Geometry: final body of the model. Coordinates: model frame, mm. A direction names the side the tool comes from. Round coordinates to 2 decimals unless told otherwise and drop trailing zeros. Write each loop counter-clockwise with the first axis right and the second up, starting at its lowest first coordinate (ties: lowest second). Pieces come first, ordered by that corner, then holes. Notation, with made-up numbers: M 65.25,-5.75 L 85.25,-5.75 A26 cw 85.25,17.25 Z; hole C 68,44.5 d3. An arc over 180 degrees is marked long. Answer as CSV lines item,"result". Start each with the question number.
Q1. Section query A-A on y = -38. Output: boundary loops of the cut face in (x, z), and give its area (3 significant figures).
Q2. Mould query, pull axis X, two halves, no side actions, for faces 3 (the cylindrical face through (18.783, -0.661, 5.037)), 4 (the flat face through (0, -1, -6)), 5 (the flat face through (-5.08, -1, -8)). Classes: pulls with the +X half, pulls with the -X half, needs draft (parallel to the pull), parting line crosses it, or undercut.
Q3. Ray query, probe 1 along Y at (x, z) = (-46.5, -3); probe 2 along Z at (x, y) = (-28, 38); probe 3 along Y at (x, z) = (-25, -7.5). Return the intervals inside material, ascending.
Q4. Reachability of faces 1 (the flat face through (-131, -96.52, 1)), 2 (the flat face through (-125, 101.6, 2)) from +Z, -Z, +X, -X, +Y, -Y: full face, straight path, thin tool, end or side. Return the list, or none.
Q5. Section query B-B on y = 0. Output: boundary loops of the cut face in (x, z), and give its area (3 significant figures).
Q6. First-contact query: pin 1 (2 mm diameter, centred on x = -151, y = 44, fed in from +Z); pin 2 (8 mm diameter, centred on x = -267.5, y = 29.5, fed in from -Z); pin 3 (1.5 mm diameter, centred on x = -265.5, y = -12, fed in from -Z). Flat tips, straight axial feed; report the tip coordinate or a pass-through.
```python
from build123d import *

# Parameters (mm, degrees)
F2_DEPTH     = 101.6
F3_T         = -5.08
F0_R         = 5.08
F4_DEPTH     = 38.1
F5_T4_DEPTH  = 134.2759536589
F5_S5_R      = 576.6246219757
F5_T6_DEPTH  = 71
F5_T10_DEPTH = 134.2759536589
F5_S11_R     = 576.6246219757
F5_T12_DEPTH = 71
F5_T13_DEPTH = 202.727744005
F6_R         = 12.7
F7_R         = 5.08


# Not quite as in the source:
# - a fillet or chamfer that OpenCascade refuses, or shapes differently, is made with other operations: its cross-section is extruded or revolved along the edge and cut away or added


with BuildPart() as f2:
    # F1 (on Front) → F2 (new body, symmetric)
    with BuildSketch(Plane.XZ):
        with BuildLine():
            Line((0, -49.880515784), (0, 25.847228221))
            Line((0, 25.847228221), (-304.8, 25.847228221))
            ThreePointArc((-304.8, 25.847228221), (-157.6074099904, -32.9761822695), (0, -49.880515784))
        make_face()
    extrude(amount=F2_DEPTH, both=True)

    # F3
    f3_openings = [f2.faces().sort_by_distance(p)[0] for p in [
        (-152.4, 0, 25.847228),
    ]]
    offset(amount=F3_T, openings=f3_openings)

    # F0 (on Right) → F4 (join)
    with BuildSketch(Plane.YZ):
        Circle(F0_R)
    extrude(amount=F4_DEPTH)

    # F5: fillet of radius 25.4 on 4 edges, made by hand


with BuildPart() as f5_tool2:
    # F5_s3 → F5_t4 (new body)
    with BuildSketch(Plane.XY.offset(25.847228221)):
        with BuildLine():
            ThreePointArc((-5.08, -71.12), (-12.5194877579, -89.0805122421), (-30.48, -96.52))
            Line((-30.48, -96.52), (-5.08, -96.52))
            Line((-5.08, -96.52), (-5.08, -71.12))
        make_face()
    extrude(amount=-F5_T4_DEPTH)

    # F5_s5 → F5_t6 (intersect, symmetric)
    with BuildSketch(Plane.XZ.offset(83.8)):
        with Locations((-17.3467118203, 531.5654050176)):
            Circle(F5_S5_R)
    extrude(amount=F5_T6_DEPTH, both=True, mode=Mode.INTERSECT)


with BuildPart() as f2_1:
    add(f2.part)

    # F5_t1: union F5_tool2
    add(f5_tool2.part)


with BuildPart() as f5_tool8:
    # F5_s9 → F5_t10 (new body)
    with BuildSketch(Plane.XY.offset(25.847228221)):
        with BuildLine():
            ThreePointArc((-30.48, 96.52), (-12.5194877579, 89.0805122421), (-5.08, 71.12))
            Line((-5.08, 71.12), (-5.08, 96.52))
            Line((-5.08, 96.52), (-30.48, 96.52))
        make_face()
    extrude(amount=-F5_T10_DEPTH)

    # F5_s11 → F5_t12 (intersect, symmetric)
    with BuildSketch(Plane.XZ.offset(-83.8)):
        with Locations((-17.3467118203, 531.5654050176)):
            Circle(F5_S11_R)
    extrude(amount=F5_T12_DEPTH, both=True, mode=Mode.INTERSECT)


with BuildPart() as f2_2:
    add(f2_1.part)

    # F5_t7: union F5_tool8
    add(f5_tool8.part)

    # F5_s14 → F5_t13 (cut)
    with BuildSketch(Plane.XY.offset(-113.380515784)):
        with BuildLine():
            ThreePointArc((0, -76.2), (-7.4394877579, -94.1605122421), (-25.4, -101.6))
            Line((-25.4, -101.6), (0, -101.6))
            Line((0, -101.6), (0, -76.2))
        make_face()
        with BuildLine():
            ThreePointArc((0, 76.2), (-7.4394877579, 94.1605122421), (-25.4, 101.6))
            Line((-25.4, 101.6), (0, 101.6))
            Line((0, 101.6), (0, 76.2))
        make_face()
    extrude(amount=F5_T13_DEPTH, mode=Mode.SUBTRACT)

    # F6
    f6_edges = [f2_2.edges().sort_by_distance(p)[0] for p in [
        (-7.439388, -94.160412, -50.054842),
        (0, 0, -49.880516),
        (-169.899659, -101.6, -29.779289),
        (-5.918318, 92.497978, -50.026943),
        (-169.899659, 101.6, -29.779289),
    ]]
    fillet(f6_edges, radius=F6_R)

    # F7
    f7_edges = [f2_2.edges().sort_by_distance(p)[0] for p in [
        (-166.679144, -96.52, -25.386819),
        (-10.998525, -87.418225, -45.024272),
        (-5.08, 0, -44.928725),
        (-11.01893, 87.442584, -45.024496),
        (-166.679144, 96.52, -25.386819),
    ]]
    fillet(f7_edges, radius=F7_R)


solid = f2_2.part
```
Entries:
1,outline,"M -304.8,25.85 A581.7 ccw -12.6,-50.12 A12.7 ccw 0,-37.42 L 0,25.85 L -5.08,25.85 L -5.08,-39.93 A5.08 cw -10.1,-45.01 A576.62 cw -294.38,25.85 Z"
1,area,"1,920 mm^2"
2,face 3,"needs draft"
2,face 4,"pulls with the +X half"
2,face 5,"undercut"
3,probe 1,"y = -101.6 to -96.52, 96.52 to 101.6"
3,probe 2,"z = -50.04 to -44.96"
3,probe 3,"y = -101.6 to -95.92, 95.92 to 101.6"
4,face 1,"+Z"
4,face 2,"+Z, -Z, +X, -X, +Y"
5,outline,"M -304.8,25.85 A581.7 ccw -12.6,-50.12 A12.7 ccw 0,-37.42 L 0,-5.08 L 38.1,-5.08 L 38.1,5.08 L 0,5.08 L 0,25.85 L -5.08,25.85 L -5.08,-39.93 A5.08 cw -10.1,-45.01 A576.62 cw -294.38,25.85 Z"
5,area,"2,300 mm^2"
6,pin 1,"stops at z = -29.12"
6,pin 2,"stops at z = 4.51"
6,pin 3,"stops at z = 5.09"
